CAD build for the part. Positions are in the model's coordinates, mm. A direction names the side the tool comes from. Give positions to 0.01 mm unless a question says otherwise; leave off trailing zeros. Loops run counter-clockwise (first coordinate to the right, second up) from the corner with the lowest first, then second, coordinate; pieces in that order, holes last.
Item 1: Mould opens along X. For faces 3 (the flat face through (135.975, 119.719, 12.098)), 4 (the flat face through (180, 89, 9)), 5 (the flat face through (89, 0, 9)), 6 (the flat face through (90, 36, 5)) say: released by +X, released by -X, zero draft, split by the parting line, or undercut.
Item 2: Drop flat-ended pins along their axis: P1, Ø10.5, axis at x = 73, y = 47.5, coming from the +Z side; P2, Ø1.6, axis at x = 138, y = 92, coming from the +Z side. Give the stop position or say it passes through.
Item 3: Which spindle directions (+Z, -Z, +X, -X, +Y, -Y) get a long thin tool onto all of the face, cutting with end or side? Do faces 1 (the cylindrical face through (29.626, 124.927, 12.098)), 2 (the cylindrical face through (173.986, 5.703, 9.367)). Say none if no direction does.
Item 4: Probe probe 1 along X at (y, z) = (92.5, 17.75); probe 2 along Y at (x, z) = (129, 12.25); probe 3 along X at (y, z) = (155.5, 17.5). List the from-to ranges inside material, lowest first.
Item 5: Saw through at B-B on y = 111. Give the cut face in (x, z), plus the area to 4 significant figures.
Item 6: Saw through at C-C on z = 15.75. Give the number of separate pieces and of enclosed holes in the cut face, plus the area to 3 significant figures.
Item 7: Saw through at A-A on y = 26.5. Give the cut face in (x, z), plus the area to 3 significant figures.
from build123d import *

# Parameters (mm, degrees)
F1_DEPTH = 19
F5_DEPTH = 19.001
F6_DEPTH = 14
F7_R     = 5


with BuildPart() as f1:
    # F0 (on Top) → F1 (new body)
    with BuildSketch(Plane.XY):
        with BuildLine():
            ThreePointArc((0, 20), (5.857864, 5.857864), (20, 0))
            Line((20, 0), (160, 0))
            ThreePointArc((160, 0), (174.142136, 5.857864), (180, 20))
            Line((180, 20), (180, 160))
            ThreePointArc((180, 160), (174.142136, 174.142136), (160, 180))
            Line((160, 180), (20, 180))
            ThreePointArc((20, 180), (5.857864, 174.142136), (0, 160))
            Line((0, 160), (0, 20))
        make_face()
    extrude(amount=F1_DEPTH)

    # F4 (on face) → F5 (cut, through all)
    with BuildSketch(Plane.XY.offset(19)):
        with BuildLine():
            ThreePointArc((124.022427, 81.785714), (120.310889, 107.5), (99.897433, 123.571429))
            ThreePointArc((99.897433, 123.571429), (96.546537, 117.440711), (90, 115))
            ThreePointArc((90, 115), (83.453463, 117.440711), (80.102567, 123.571429))
            ThreePointArc((80.102567, 123.571429), (59.689111, 107.5), (55.977573, 81.785714))
            ThreePointArc((55.977573, 81.785714), (62.962379, 81.949112), (68.349365, 77.5))
            ThreePointArc((68.349365, 77.5), (69.508916, 70.610178), (65.875007, 64.642857))
            ThreePointArc((65.875007, 64.642857), (90, 55), (114.124993, 64.642857))
            ThreePointArc((114.124993, 64.642857), (110.491084, 70.610178), (111.650635, 77.5))
            ThreePointArc((111.650635, 77.5), (117.037621, 81.949112), (124.022427, 81.785714))
        make_face()
    extrude(amount=-F5_DEPTH, mode=Mode.SUBTRACT)

    # F2 (on face) + F3 (on face) → F6 (cut)
    with BuildSketch(Plane.XY.offset(19)):
        with BuildLine():
            ThreePointArc((45.05304, 105), (42.30304, 107.75), (39.55304, 105))
            Line((39.55304, 105), (39.55304, 75))
            ThreePointArc((39.55304, 75), (42.30304, 72.25), (45.05304, 75))
            Line((45.05304, 75), (45.05304, 105))
        make_face()
        with BuildLine():
            ThreePointArc((51.786139, 126.188349), (50.779569, 122.431779), (54.536139, 121.425209))
            Line((54.536139, 121.425209), (80.516901, 136.425209))
            ThreePointArc((80.516901, 136.425209), (81.523471, 140.181779), (77.766901, 141.188349))
            Line((77.766901, 141.188349), (51.786139, 126.188349))
        make_face()
        with BuildLine():
            ThreePointArc((102.233099, 141.188349), (98.476529, 140.181779), (99.483099, 136.425209))
            Line((99.483099, 136.425209), (125.463861, 121.425209))
            ThreePointArc((125.463861, 121.425209), (129.220431, 122.431779), (128.213861, 126.188349))
            Line((128.213861, 126.188349), (102.233099, 141.188349))
        make_face()
        with BuildLine():
            ThreePointArc((140.44696, 105), (137.69696, 107.75), (134.94696, 105))
            Line((134.94696, 105), (134.94696, 75))
            ThreePointArc((134.94696, 75), (137.69696, 72.25), (140.44696, 75))
            Line((140.44696, 75), (140.44696, 105))
        make_face()
        with BuildLine():
            ThreePointArc((128.213861, 53.811651), (129.220431, 57.568221), (125.463861, 58.574791))
            Line((125.463861, 58.574791), (99.483099, 43.574791))
            ThreePointArc((99.483099, 43.574791), (98.476529, 39.818221), (102.233099, 38.811651))
            Line((102.233099, 38.811651), (128.213861, 53.811651))
        make_face()
        with BuildLine():
            ThreePointArc((77.766901, 38.811651), (81.523471, 39.818221), (80.516901, 43.574791))
            Line((80.516901, 43.574791), (54.536139, 58.574791))
            ThreePointArc((54.536139, 58.574791), (50.779569, 57.568221), (51.786139, 53.811651))
            Line((51.786139, 53.811651), (77.766901, 38.811651))
        make_face()
    with BuildSketch(Plane.XY.offset(19)):
        with BuildLine():
            ThreePointArc((87.25, 23), (90, 20.25), (92.75, 23))
            Line((92.75, 23), (92.75, 48))
            ThreePointArc((92.75, 48), (90, 50.75), (87.25, 48))
            Line((87.25, 48), (87.25, 23))
        make_face()
        with BuildLine():
            ThreePointArc((30.601298, 58.88157), (29.594728, 55.125), (33.351298, 54.11843))
            Line((33.351298, 54.11843), (55.001933, 66.61843))
            ThreePointArc((55.001933, 66.61843), (56.008503, 70.375), (52.251933, 71.38157))
            Line((52.251933, 71.38157), (30.601298, 58.88157))
        make_face()
        with BuildLine():
            ThreePointArc((33.351298, 125.88157), (29.594728, 124.875), (30.601298, 121.11843))
            Line((30.601298, 121.11843), (52.251933, 108.61843))
            ThreePointArc((52.251933, 108.61843), (56.008503, 109.625), (55.001933, 113.38157))
            Line((55.001933, 113.38157), (33.351298, 125.88157))
        make_face()
        with BuildLine():
            ThreePointArc((92.75, 157), (90, 159.75), (87.25, 157))
            Line((87.25, 157), (87.25, 132))
            ThreePointArc((87.25, 132), (90, 129.25), (92.75, 132))
            Line((92.75, 132), (92.75, 157))
        make_face()
        with BuildLine():
            ThreePointArc((149.398702, 121.11843), (150.405272, 124.875), (146.648702, 125.88157))
            Line((146.648702, 125.88157), (124.998067, 113.38157))
            ThreePointArc((124.998067, 113.38157), (123.991497, 109.625), (127.748067, 108.61843))
            Line((127.748067, 108.61843), (149.398702, 121.11843))
        make_face()
        with BuildLine():
            ThreePointArc((146.648702, 54.11843), (150.405272, 55.125), (149.398702, 58.88157))
            Line((149.398702, 58.88157), (127.748067, 71.38157))
            ThreePointArc((127.748067, 71.38157), (123.991497, 70.375), (124.998067, 66.61843))
            Line((124.998067, 66.61843), (146.648702, 54.11843))
        make_face()
    extrude(amount=-F6_DEPTH, mode=Mode.SUBTRACT)

    # F7
    f7_edges = [f1.edges().sort_by_distance(p)[0] for p in [
        (80.102567, 123.571429, 9.5),
        (99.897433, 123.571429, 9.5),
        (55.977573, 81.785714, 9.5),
        (65.875007, 64.642857, 9.5),
        (114.124993, 64.642857, 9.5),
        (124.022427, 81.785714, 9.5),
    ]]
    fillet(f7_edges, radius=F7_R)


solid = f1.part
Results below:
1. face 3: undercut
1. face 4: released by +X
1. face 5: zero draft
1. face 6: undercut
2. P1: stops at z = 19
2. P2: stops at z = 5
3. face 1: +Z
3. face 2: +Z, -Z, +X, -Y
4. probe 1: x = 0 to 39.55, 45.05 to 55.09, 124.91 to 134.95, 140.45 to 180
4. probe 2: y = 0 to 54.49, 57.89 to 64.31, 70.66 to 109.34, 115.69 to 122.11, 125.51 to 180
4. probe 3: x = 0 to 87.25, 92.75 to 180
5. outline: (0, 0) - (62, 0) - (62, 19) - (56.38, 19) - (56.38, 5) - (48.13, 5) - (48.13, 19) - (0, 19) - close; (118, 0) - (180, 0) - (180, 19) - (131.87, 19) - (131.87, 5) - (123.62, 5) - (123.62, 19) - (118, 19) - close
5. area: 2,125 mm2
6. separate pieces: 1
6. enclosed holes: 13
6. area: 26,600 mm2
7. outline: (0, 0) - (180, 0) - (180, 19) - (92.75, 19) - (92.75, 5) - (87.25, 5) - (87.25, 19) - (0, 19) - close
7. area: 3,340 mm2
